Read the model definition and answer for the solid it produces. Units are mm, in the model's axes. Give positions to 0.01 mm unless a question says otherwise; leave off trailing zeros. Order: outer loops, then holes, each group sorted by start corner. A loop starts at its lowest first (then second) coordinate and runs counter-clockwise, first axis right, second up. Notation, with made-up numbers: M 20,7 L 28,7 A26 cw 28,23 Z; hole C -26,-24 d7. An arc over 180 degrees is marked long. One line per item, written item: value.
Autodesk Fusion 360 part; units mm, degrees
sketch "Sketch1" plane through (0, 0, 0) normal (0, 0, 1) x (1, 0, 0)
  circle A0 centre (0, 0) radius 1.65
  circle A1 centre (0, 0) radius 7.5
  dimension "d1" = 3.3
  dimension "d2" = 15
extrude "Extrude1" add sketch "Sketch1" along normal blind 25
chamfer "Chamfer1" distance 0.5 angle 45 2 faces at (5.5159, -0.4546, 25) (5.5159, -0.4546, 0)
1) Find section C-C, the plane z = 2. Write down the section's boundary in (x, y).
Reported:
outline: C 0,0 d15; hole C 0,0 d3.3
2) Each of these flat-tipped pins is pushed along its axis until it touches: pin 1 Ø4 at (x, z) = (-2.5, 15.5) entering from +Y; pin 2 Ø2.5 at (x, y) = (0, 0) entering from +Z; pin 3 Ø6 at (x, z) = (-3.5, 22) entering from -Y; pin 4 Ø6 at (x, z) = (5.5, 5) entering from -Y. Where does it stop, or does it pass through?
Reported:
pin 1: stops at y = 7.48
pin 2: passes through
pin 3: stops at y = -7.48
pin 4: stops at y = -7.07
3) Consider probe 1 along Y at (x, z) = (0, 16.5); probe 2 along X at (y, z) = (1.5, 19); probe 3 along X at (y, z) = (-0.5, 4.25). Determine where each line is inside the solid, lowest interval first.
Reported:
probe 1: y = -7.5 to -1.65, 1.65 to 7.5
probe 2: x = -7.35 to -0.69, 0.69 to 7.35
probe 3: x = -7.48 to -1.57, 1.57 to 7.48
4) Find section A-A, the plane x = 0. Write down the section's boundary in (y, z).
Reported:
outline: M -7.5,0.5 L -7,0 L -2.15,0 L -1.65,0.5 L -1.65,24.5 L -2.15,25 L -7,25 L -7.5,24.5 Z; M 1.65,0.5 L 2.15,0 L 7,0 L 7.5,0.5 L 7.5,24.5 L 7,25 L 2.15,25 L 1.65,24.5 Z
5) Determine the mould class of faces 1 (the face through (-7.493, -0.33, 12.332)), 2 (the face through (-1.216, -1.115, 12.332)), 3 (the face through (-2, 2, 25)) for opening direction Y: +Y half, -Y half, draft (parallel to the pull), parting line (faces both ways), or undercut.
Reported:
face 1: parting line
face 2: undercut
face 3: draft
